Check sheet for the drawn part. Datum: minimum x, y, z corner. Units: mm. A direction names the side the tool comes from. Give positions to 0.01 mm unless a question says otherwise; leave off trailing zeros. Loops run counter-clockwise (first coordinate to the right, second up) from the corner with the lowest first, then second, coordinate; pieces in that order, holes last. Notation, with made-up numbers: (71, 45) - (110, 45) arc R23 ccw to (110, 81) - close; hole circle Ø8 at (0, 21). An arc over 180 degrees is marked (long way). Answer in a Markdown table with one row per item.
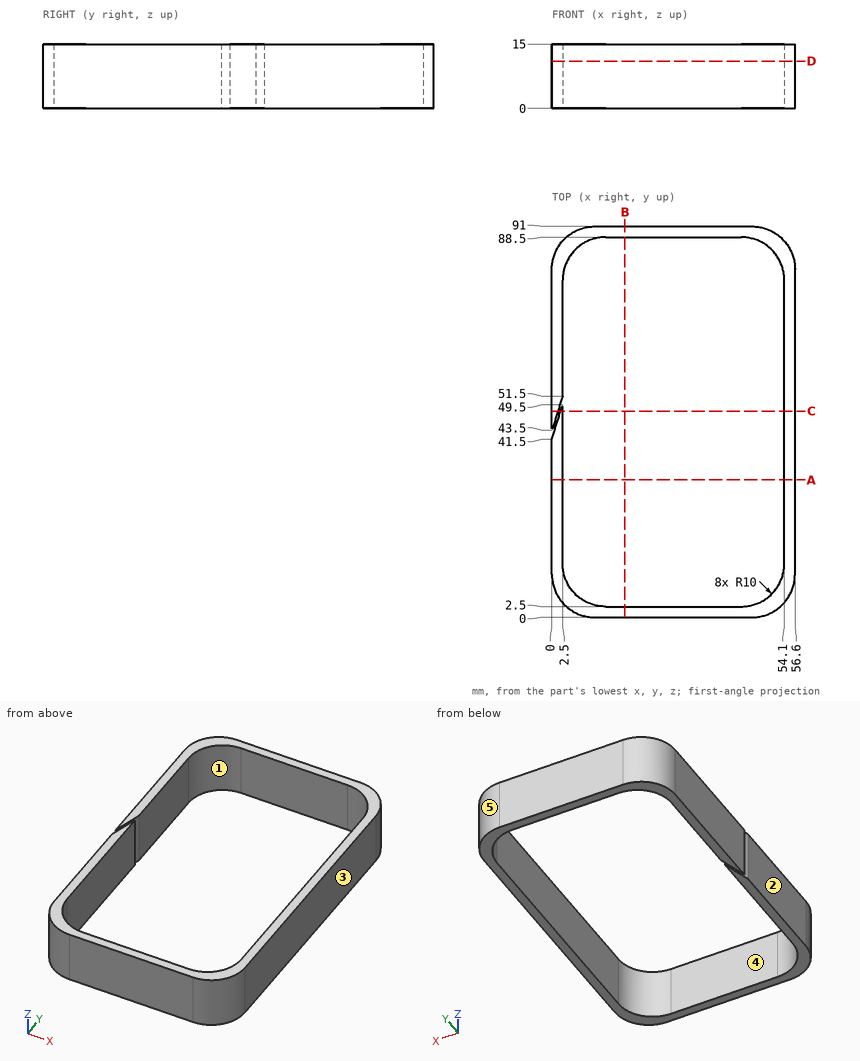
Q1. Sectioned sample at D-D (z = 11). Record the cut outline in (x, y).
Completed:
| item | result |
|---|---|
| outline | (0, 10) arc R10 ccw to (10, 0) - (46.6, 0) arc R10 ccw to (56.6, 10) - (56.6, 81) arc R10 ccw to (46.6, 91) - (10, 91) arc R10 ccw to (0, 81) - (0, 43.5) - (2.5, 51.5) - (2.5, 78.5) arc R10 cw to (12.5, 88.5) - (44.1, 88.5) arc R10 cw to (54.1, 78.5) - (54.1, 12.5) arc R10 cw to (44.1, 2.5) - (12.5, 2.5) arc R10 cw to (2.5, 12.5) - (2.5, 49.5) - (0, 41.5) - close |
Q2. Draft check along Y on the marked faces 3, 4 and 5. Enter one of: +Y half, -Y half, draft (parallel to the pull), parting line (faces both ways), or undercut.
Completed:
| item | result |
|---|---|
| face 3 | draft |
| face 4 | undercut |
| face 5 | +Y half |
Q3. Sectioned sample at C-C (y = 48). Record the cut outline in (x, z).
Completed:
| item | result |
|---|---|
| outline | (0, 0) - (1.41, 0) - (1.41, 15) - (0, 15) - close; (2.03, 0) - (2.5, 0) - (2.5, 15) - (2.03, 15) - close; (54.1, 0) - (56.6, 0) - (56.6, 15) - (54.1, 15) - close |
Q4. Tool access check on the marked faces 1 and 2. Record the directions out of +Z, -Z, +X, -X, +Y, -Y that give a thin tool (end or side, any length) a straight path to the whole face; none if there is none.
Completed:
| item | result |
|---|---|
| face 1 | +Z, -Z |
| face 2 | +Z, -Z, -X, +Y, -Y |
Q5. Sectioned sample at A-A (y = 32). Record the cut outline in (x, z), and give its area (3 significant figures).
Completed:
| item | result |
|---|---|
| outline | (0, 0) - (2.5, 0) - (2.5, 15) - (0, 15) - close; (54.1, 0) - (56.6, 0) - (56.6, 15) - (54.1, 15) - close |
| area | 75.0 mm^2 |
Q6. Go/stop test with a flat-tipped pin: P1, Ø6, axis at x = 17, z = 5, coming from the -Y side. Record where the tip stops, or that it passes through.
Completed:
| item | result |
|---|---|
| P1 | y = 0 |
Q7. Sectioned sample at B-B (x = 17). Record the cut outline in (y, z), and give its area (3 significant figures).
Completed:
| item | result |
|---|---|
| outline | (0, 0) - (2.5, 0) - (2.5, 15) - (0, 15) - close; (88.5, 0) - (91, 0) - (91, 15) - (88.5, 15) - close |
| area | 75.0 mm^2 |
Q8. Thickness scan on line 1 (Y direction, x = 24.5, z = 12); line 2 (X direction, y = 74.5, z = 8); line 3 (X direction, y = 81, z = 9.25). Record the ranges inside material, lowest first.
Completed:
| item | result |
|---|---|
| line 1 | 0 to 2.5, 88.5 to 91 |
| line 2 | 0 to 2.5, 54.1 to 56.6 |
| line 3 | 0 to 2.82, 53.78 to 56.6 |
